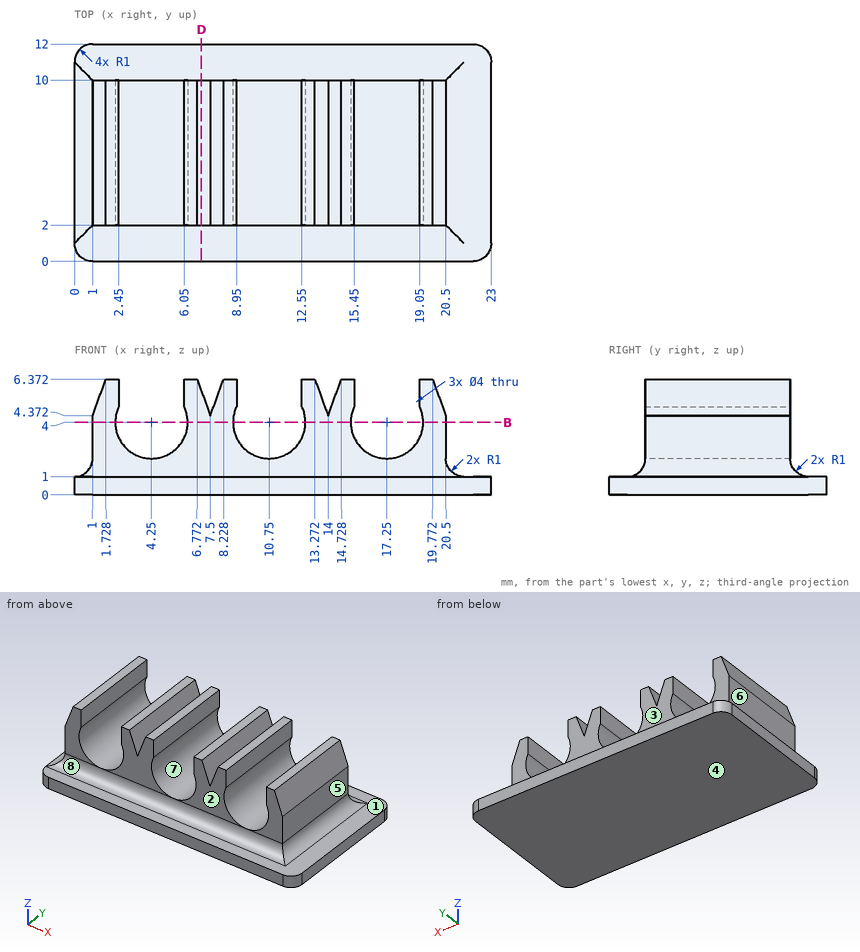
Could you check a few things on this drawing? It's one solid part, dimensions in mm from its lowest x, y, z. A direction names the side the tool comes from. Coordinates: 2 decimals unless noted, no trailing zeros. Write each loop counter-clockwise with the first axis right and the second up, starting at its lowest first coordinate (ties: lowest second). Pieces come first, ordered by that corner, then holes.
Q1. Imagine slicing it at B-B, the plane z = 4. List the corners of the cut face in (x, y) for me, plus the area to 3 significant figures.
Results found:
outline: (1, 2) - (2.25, 2) - (2.25, 10) - (1, 10) - close; (6.25, 2) - (8.75, 2) - (8.75, 10) - (6.25, 10) - close; (12.75, 2) - (15.25, 2) - (15.25, 10) - (12.75, 10) - close; (19.25, 2) - (20.5, 2) - (20.5, 10) - (19.25, 10) - close
area: 60.0 mm2
Q2. For P1, Ø2, axis at x = 12.5, z = 3.5, coming from the +Y side; P2, Ø0.7, axis at y = 7.5, z = 3, coming from the -X side; P3, Ø1.5, axis at x = 14.5, y = 9.5, coming from the +Z side; P4, Ø1.5, axis at y = 9.5, z = 2, coming from the -X side, each with a flat end and sliding along its axis, tell me the tip position at first contact or that it passes through.
Results found:
P1: stops at y = 10
P2: stops at x = 1
P3: stops at z = 6.37
P4: stops at x = 0.66
Q3. If we mould it in two halves opening along X, with no side actions, what happens to the marked faces 6, 7 and 8? For each: +X half, -X half, draft (parallel to the pull), parting line (faces both ways), or undercut.
Results found:
face 6: -X half
face 7: undercut
face 8: draft
Q4. Imagine slicing it at D-D, the plane x = 7. List the corners of the cut face in (y, z) for me, plus the area to 3 significant figures.
Results found:
outline: (0, 0) - (12, 0) - (12, 1) - (11, 1) arc R1 cw to (10, 2) - (10, 5.75) - (2, 5.75) - (2, 2) arc R1 cw to (1, 1) - (0, 1) - close
area: 50.4 mm2
Q5. Which directions (+Z, -Z, +X, -X, +Y, -Y) give clear straight access to the entire face, cutting with the end or side of a thin tool? Please do the marked faces 1, 2, 3, 4 and 5.
Results found:
face 1: +Z, +X
face 2: +Z, +X, -X, -Y
face 3: +Z, +X, -X, +Y
face 4: -Z, +X, -X, +Y, -Y
face 5: +Z, +X, +Y, -Y
Q6. Please list where these lines run through material, in increasing order: L1, parallel to X at y = 8, z = 4; L2, parallel to X at y = 6.25, z = 3; L3, parallel to Y at x = 6.5, z = 5.5.
Results found:
L1: x = 1 to 2.25, 6.25 to 8.75, 12.75 to 15.25, 19.25 to 20.5
L2: x = 1 to 2.52, 5.98 to 9.02, 12.48 to 15.52, 18.98 to 20.5
L3: y = 2 to 10
